Source: CAD feature listing. Evaluate the final solid. Frame: model axes, mm. A direction names the side the tool comes from. Give positions to 0.01 mm unless a question says otherwise; leave off trailing zeros. Loops run counter-clockwise (first coordinate to the right, second up) from the corner with the lowest first, then second, coordinate; pieces in that order, holes last. Notation, with made-up numbers: (9, 48) -> (47, 48) arc R9 cw to (47, 54) -> close; hole circle Ø1 at (-8.75, -36.5). An arc over 180 degrees is marked (long way). Return JSON: item names as keys, results as strings. Group by question number.
(1) Cut plane D-D on x = -25. Return loops of the section in (y, z).
(2) Cut plane A-A on x = -51. Return loops of the section in (y, z), then the cut area to 3 significant figures.
(3) Ray query, line 1 (Z direction, x = -75, y = 0.75); line 2 (Z direction, x = -39, y = 1); line 3 (Z direction, x = 6, y = 0.7). Return the intervals inside material, ascending. Write a range as from..to.
(4) Cut plane B-B on z = 50. Return loops of the section in (x, y).
(5) Draft query along X for faces 3 (the face through (-9.474, 0.986, 51.669)), 4 (the face through (51.99, 0.99, 52.15)), 5 (the face through (2, 0, -1)). Return one class per face: released by +X, released by -X, zero draft, split by the parting line, or undercut.
(6) Cut plane C-C on x = 10. Give the number of separate pieces and of enclosed holes in the cut face, then the cut area to 3 significant figures.
(7) Access query for faces 1 (the face through (-40.365, 0.986, 35.415)), 2 (the face through (-52.15, 0.99, 51.99)). Directions: +Z, -Z, +X, -X, +Y, -Y. A direction counts if a zero-diameter tool reaches every point of the face in a straight line with its end or side. Return the directions, or none.
```python
from build123d import *

# Parameters (mm, degrees)
SKETCH_1_R      = 1.75
EXTRUDE_1_DEPTH = 2


with BuildPart() as part:
    # 草图1 → 凸台-拉伸1 (new body)
    with BuildSketch(Plane(origin=(0, 0, 0), x_dir=(1, 0, 0), z_dir=(0, 1, 0))):
        with BuildLine():
            Line((-45, -55), (45, -55))
            ThreePointArc((45, -55), (52.071067812, -52.071067812), (55, -45))
            Line((55, -45), (55, 45))
            ThreePointArc((55, 45), (52.071067812, 52.071067812), (45, 55))
            Line((45, 55), (-45, 55))
            ThreePointArc((-45, 55), (-52.071067812, 52.071067812), (-55, 45))
            Line((-55, 45), (-55, 19.989791925))
            ThreePointArc((-55, 19.989791925), (-56.465368542, 16.453355802), (-60.002552182, 14.989792577))
            Line((-60.002552182, 14.989792577), (-74.997444562, 14.997446515))
            ThreePointArc((-74.997444562, 14.997446515), (-78.534628201, 13.53388329), (-79.999996743, 9.997447167))
            Line((-79.999996743, 9.997447167), (-79.999996743, -9.997447167))
            ThreePointArc((-79.999996743, -9.997447167), (-78.534628201, -13.53388329), (-74.997444562, -14.997446515))
            Line((-74.997444562, -14.997446515), (-60.002552182, -14.989792577))
            ThreePointArc((-60.002552182, -14.989792577), (-56.465368542, -16.453355802), (-55, -19.989791925))
            Line((-55, -19.989791925), (-55, -45))
            ThreePointArc((-55, -45), (-52.071067812, -52.071067812), (-45, -55))
        make_face()
        with Locations(Location((-45.961940777, -45.961940777, 0), (0, 0, 270))):
            Circle(SKETCH_1_R, mode=Mode.SUBTRACT)
        with Locations(Location((-75, -10, 0), (0, 0, 270))):
            Circle(SKETCH_1_R, mode=Mode.SUBTRACT)
        with Locations(Location((-51, -10, 0), (0, 0, 270))):
            Circle(SKETCH_1_R, mode=Mode.SUBTRACT)
        with BuildLine():
            Line((-45, 40.050252532), (-35.857864376, 30.908116908))
            ThreePointArc((-35.857864376, 30.908116908), (-31.52240935, 24.419649932), (-30, 16.765981284))
            Line((-30, 16.765981284), (-30, -16.765981284))
            ThreePointArc((-30, -16.765981284), (-31.52240935, -24.419649932), (-35.857864376, -30.908116908))
            Line((-35.857864376, -30.908116908), (-45, -40.050252532))
            Line((-45, -40.050252532), (-45, 40.050252532))
        make_face(mode=Mode.SUBTRACT)
        with Locations(Location((-10, -50, 0), (0, 0, 270))):
            Circle(SKETCH_1_R, mode=Mode.SUBTRACT)
        with Locations(Location((10, -50, 0), (0, 0, 270))):
            Circle(SKETCH_1_R, mode=Mode.SUBTRACT)
        with BuildLine():
            Line((-40.050252532, -45), (-30.908116908, -35.857864376))
            ThreePointArc((-30.908116908, -35.857864376), (-24.419649932, -31.52240935), (-16.765981284, -30))
            Line((-16.765981284, -30), (16.765981284, -30))
            ThreePointArc((16.765981284, -30), (24.419649932, -31.52240935), (30.908116908, -35.857864376))
            Line((30.908116908, -35.857864376), (40.050252532, -45))
            Line((40.050252532, -45), (-40.050252532, -45))
        make_face(mode=Mode.SUBTRACT)
        with Locations(Location((45.961940777, -45.961940777, 0), (0, 0, 270))):
            Circle(SKETCH_1_R, mode=Mode.SUBTRACT)
        Polygon((0, -4.32233047), (17.67766953, -22), (-17.67766953, -22), align=None, mode=Mode.SUBTRACT)
        with Locations(Location((50, -10, 0), (0, 0, 270))):
            Circle(SKETCH_1_R, mode=Mode.SUBTRACT)
        with Locations(Location((-75, 10, 0), (0, 0, 270))):
            Circle(SKETCH_1_R, mode=Mode.SUBTRACT)
        with Locations(Location((-51, 10, 0), (0, 0, 270))):
            Circle(SKETCH_1_R, mode=Mode.SUBTRACT)
        with Locations(Location((-25, 0, 0), (0, 0, 270))):
            Circle(SKETCH_1_R, mode=Mode.SUBTRACT)
        Polygon((-4.32233047, 0), (-22, -17.67766953), (-22, 17.67766953), align=None, mode=Mode.SUBTRACT)
        with Locations(Location((-45.961940777, 45.961940777, 0), (0, 0, 270))):
            Circle(SKETCH_1_R, mode=Mode.SUBTRACT)
        Polygon((0, 4.32233047), (-17.67766953, 22), (17.67766953, 22), align=None, mode=Mode.SUBTRACT)
        Polygon((4.32233047, 0), (22, 17.67766953), (22, -17.67766953), align=None, mode=Mode.SUBTRACT)
        with Locations(Location((25, 0, 0), (0, 0, 270))):
            Circle(SKETCH_1_R, mode=Mode.SUBTRACT)
        with BuildLine():
            Line((45, -40.050252532), (35.857864376, -30.908116908))
            ThreePointArc((35.857864376, -30.908116908), (31.52240935, -24.419649932), (30, -16.765981284))
            Line((30, -16.765981284), (30, 16.765981284))
            ThreePointArc((30, 16.765981284), (31.52240935, 24.419649932), (35.857864376, 30.908116908))
            Line((35.857864376, 30.908116908), (45, 40.050252532))
            Line((45, 40.050252532), (45, -40.050252532))
        make_face(mode=Mode.SUBTRACT)
        with Locations(Location((50, 10, 0), (0, 0, 270))):
            Circle(SKETCH_1_R, mode=Mode.SUBTRACT)
        with BuildLine():
            ThreePointArc((-16.765981284, 30), (-24.419649932, 31.52240935), (-30.908116908, 35.857864376))
            Line((-30.908116908, 35.857864376), (-40.050252532, 45))
            Line((-40.050252532, 45), (40.050252532, 45))
            Line((40.050252532, 45), (30.908116908, 35.857864376))
            ThreePointArc((30.908116908, 35.857864376), (24.419649932, 31.52240935), (16.765981284, 30))
            Line((16.765981284, 30), (-16.765981284, 30))
        make_face(mode=Mode.SUBTRACT)
        with Locations(Location((-10, 50, 0), (0, 0, 270))):
            Circle(SKETCH_1_R, mode=Mode.SUBTRACT)
        with Locations(Location((10, 50, 0), (0, 0, 270))):
            Circle(SKETCH_1_R, mode=Mode.SUBTRACT)
        with Locations(Location((45.961940777, 45.961940777, 0), (0, 0, 270))):
            Circle(SKETCH_1_R, mode=Mode.SUBTRACT)
    extrude(amount=EXTRUDE_1_DEPTH)


solid = part.part
```
Answers:
{
 "1": {"outline": "(0, -55) -> (2, -55) -> (2, -45) -> (0, -45) -> close; (0, -31.77) -> (2, -31.77) -> (2, -1.75) -> (0, -1.75) -> close; (0, 1.75) -> (2, 1.75) -> (2, 31.77) -> (0, 31.77) -> close; (0, 45) -> (2, 45) -> (2, 55) -> (0, 55) -> close"},
 "2": {"outline": "(0, -53) -> (2, -53) -> (2, -11.75) -> (0, -11.75) -> close; (0, -8.25) -> (2, -8.25) -> (2, 8.25) -> (0, 8.25) -> close; (0, 11.75) -> (2, 11.75) -> (2, 53) -> (0, 53) -> close", "area": "198 mm²"},
 "3": {"line 1": "-15..-11.75, -8.25..8.25, 11.75..15", "line 2": "-55..-45, -43.95..-34.05, 34.05..43.95, 45..55", "line 3": "-55..-45, -30..-22, -10.32..-1.68, 1.68..10.32, 22..30, 45..55"},
 "4": {"outline": "(-53.66, 0) -> (-11.75, 0) -> (-11.75, 2) -> (-53.66, 2) -> close; (-8.25, 0) -> (8.25, 0) -> (8.25, 2) -> (-8.25, 2) -> close; (11.75, 0) -> (53.66, 0) -> (53.66, 2) -> (11.75, 2) -> close"},
 "5": {"face 3": "undercut", "face 4": "released by +X", "face 5": "zero draft"},
 "6": {"separate pieces": "8", "enclosed holes": "0", "area": "92.6 mm²"},
 "7": {"face 1": "+Y, -Y", "face 2": "+Z, -X, +Y, -Y"}
}
